Design review of the part built by this model. Coordinates are the model's own, in mm. Coordinates: 2 decimals unless noted, no trailing zeros. Order: outer loops, then holes, each group sorted by start corner. A loop starts at its lowest first (then second) coordinate and runs counter-clockwise, first axis right, second up. Notation, with made-up numbers: M 7.5,-7 L 30.5,-7 A25 cw 30.5,30 Z; hole C 84,-16.75 d2. An arc over 180 degrees is marked long. Use CSV: the item, a comma, the result in double quotes.
```python
from build123d import *

# Parameters (mm, degrees)
SKETCH3_W          = 12.35
SKETCH3_H          = 7
CUT_EXTRUDE1_DEPTH = 10
CIRPATTERN1_COUNT  = 18


with BuildPart() as part:
    # Sketch1 → Revolve1 (revolve)
    with BuildSketch(Plane.XY, mode=Mode.PRIVATE) as revolve1_sk:
        with BuildLine():
            Line((-27.5, 16.23), (-23.995243086, 0.778791907))
            ThreePointArc((-23.995243086, 0.778791907), (-23.644032445, 0.218588427), (-23.020016456, 0))
            Line((-23.020016456, 0), (-20.318591765, 0))
            Line((-20.318591765, 0), (-20.318591765, 1.3))
            Line((-20.318591765, 1.3), (-21.981868555, 1.3))
            ThreePointArc((-21.981868555, 1.3), (-22.605884543, 1.518588427), (-22.957095185, 2.078791907))
            Line((-22.957095185, 2.078791907), (-26.166976516, 16.23))
            Line((-26.166976516, 16.23), (-27.5, 16.23))
        make_face()
    revolve(revolve1_sk.sketch.rotate(Axis((0, 12.177236693, 0), (0, -1, 0)), 270), axis=Axis((0, 12.177236693, 0), (0, -1, 0)))

    # Sketch3 → Cut-Extrude1 (cut)
    with BuildSketch(Plane(origin=(22.653076131, -5.138337708, 0), x_dir=(0.22120809279024437, 0.9752266299092242, 0), z_dir=(0.975226629909224, -0.22120809279024434, 0))):
        with Locations((13.386150755, 0)):
            Rectangle(SKETCH3_W, SKETCH3_H)
    cut_extrude1 = extrude(amount=-CUT_EXTRUDE1_DEPTH, mode=Mode.SUBTRACT)

    # CirPattern1: Cut-Extrude1 ×18 about axis
    cirpattern1_axis = Axis((0, 0, 0), (0, 1, 0))
    for i in range(1, CIRPATTERN1_COUNT):
        add(cut_extrude1.rotate(cirpattern1_axis, i * 360 / CIRPATTERN1_COUNT), mode=Mode.SUBTRACT)


solid = part.part
```
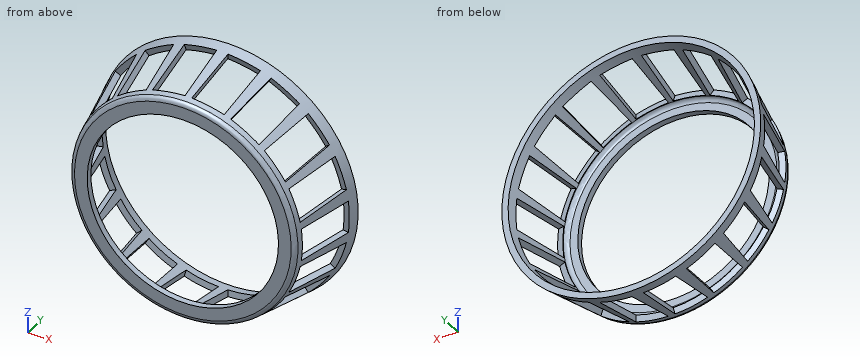
(1) Wall thickness on probe 1 along X at (y, z) = (0.65, 0); probe 2 along X at (y, z) = (8.5, -23.5); probe 3 along Z at (x, y) = (-23.5, 13): over which ranges is each line inside the solid? List them lowest first.
The answers:
probe 1,"x = -23.96 to -20.32, 20.32 to 23.96"
probe 2,"x = -9.53 to -7.7, 7.7 to 9.53"
probe 3,"z = -12.82 to -12.28, 12.28 to 12.82"
(2) Clearance check with flat-ended pins moving along their axes: P1, Ø1, axis at y = 2.5, z = -3.5, coming from the +X side; P2, Ø1.2, axis at x = 23.5, y = 7.5, coming from the -Z side; P3, Ø24.5, axis at x = 0, z = 0, coming from the -Y side; P4, Ø3, axis at x = 25.5, y = 5.5, coming from the +Z side. State where each tip first meets the part, or that it passes through.
The answers:
P1,"stops at x = 24.25"
P2,"stops at z = -5.05"
P3,"passes through"
P4,"stops at z = 5.3"
(3) Add section A-A on z = 0. State the section outline as (x, y) points.
The answers:
outline,"M -27.5,16.23 L -26.98,13.94 L -25.71,14.23 L -26.17,16.23 Z; M -24.25,1.89 L -24,0.78 A1 ccw -23.02,0 L -20.32,0 L -20.32,1.3 L -21.98,1.3 A1 cw -22.96,2.08 L -22.98,2.18 Z; M 20.32,0 L 23.02,0 A1 ccw 24,0.78 L 24.25,1.89 L 22.98,2.18 L 22.96,2.08 A1 cw 21.98,1.3 L 20.32,1.3 Z; M 25.71,14.23 L 26.98,13.94 L 27.5,16.23 L 26.17,16.23 Z"
(4) Add section B-B on x = -2.5. Give the number of separate pieces and of enclosed holes in the cut face, and give its area (3 significant figures).
The answers:
separate pieces,"4"
enclosed holes,"0"
area,"17.3 mm2"
